Design review of the part built by this model. Coordinates are the model's own, in mm. Face numbers are marked on the shaded views. A direction names the side the tool comes from. Round coordinates to 2 decimals unless told otherwise and drop trailing zeros. Write each loop counter-clockwise with the first axis right and the second up, starting at its lowest first coordinate (ties: lowest second). Pieces come first, ordered by that corner, then holes. Notation, with made-up numbers: (87, 83) -> (146, 83) arc R11 cw to (146, 94) -> close; hole circle Ø5 at (-18, 79.5). An arc over 180 degrees is marked (long way). Write item = value, one per line. Start each with the question number.
Item 1: For pin 1 Ø2 at (y, z) = (-13, 7.5) entering from +X; pin 2 Ø1.5 at (y, z) = (7.5, 10.5) entering from +X; pin 3 Ø20 at (y, z) = (-1.5, 29) entering from -X, all flat-tipped, find the tip position at first contact; note any pin that passes through.
Item 2: Machinability: for the marked faces 1, 2 and 3, which of the approach directions +Z, -Z, +X, -X, +Y, -Y give a long, thin tool a straight path to every point of the face, cutting with its end or side? Answer none if there is none.
Item 3: To check wall thickness, follow L1, parallel to Y at x = -23.5, z = 33; L2, parallel to Y at x = -42, z = 19; L3, parallel to X at y = 3.5, z = 19. State the ranges of each line that lie inside material, in increasing order.
Item 4: Add section C-C, the plane y = 27. State the section outline as (x, z) points, then the cut area to 3 significant figures.
Item 5: Add section D-D, the plane x = -37. State the section outline as (y, z) points, then the cut area to 3 significant figures.
Item 6: Add section A-A, the plane z = 25. State the section outline as (x, y) points.
Item 7: Add section B-B, the plane x = -10. State the section outline as (y, z) points, then the cut area to 3 significant figures.
Item 8: Mouldability with a two-part tool opening along Z and no side actions: class the marked faces 4, 5 and 6 as released by +Z, released by -Z, zero draft, split by the parting line, or undercut.
from build123d import *

# Parameters (mm, degrees)
SKETCH_R        = 10
PAD_DEPTH       = 35
POCKET_DEPTH    = 70.001
CHAMFER_SIZE    = 20
CHAMFER001_SIZE = 20
SKETCH002_R     = 10
POCKET001_DEPTH = 15
SKETCH003_W     = 81.266709
SKETCH003_H     = 40
POCKET002_DEPTH = 65
SKETCH004_W     = 95.373383
SKETCH004_H     = 50
POCKET003_DEPTH = 20


with BuildPart() as part:
    # Sketch → Pad (new body, symmetric)
    with BuildSketch(Plane.XZ):
        with BuildLine():
            Line((50, 50), (50, 0))
            Line((50, 0), (-50, 0))
            Line((-50, 0), (-50, 30))
            ThreePointArc((-5.278546, 50), (-29.773495, 44.772275), (-50, 30))
            Line((50, 50), (-5.278546, 50))
        make_face()
        with Locations((-10, 25)):
            Circle(SKETCH_R, mode=Mode.SUBTRACT)
    extrude(amount=PAD_DEPTH, both=True)

    # Sketch001 → Pocket (cut, through all)
    with BuildSketch(Plane.XZ.offset(35)):
        Polygon((50, 50), (30, 50), (50, 38.452995), align=None)
        Polygon((50, 0), (30, 0), (50, 11.547005), align=None)
    extrude(amount=-POCKET_DEPTH, mode=Mode.SUBTRACT)

    # Chamfer
    chamfer_edges = [part.edges().sort_by_distance(p)[0] for p in [
        (50, -35, 25),
    ]]
    chamfer(chamfer_edges, length=CHAMFER_SIZE)

    # Chamfer001
    chamfer001_edges = [part.edges().sort_by_distance(p)[0] for p in [
        (50, 35, 25),
    ]]
    chamfer(chamfer001_edges, length=CHAMFER001_SIZE)

    # Sketch002 → Pocket001 (cut)
    with BuildSketch(Plane(origin=(50, 0, 0), x_dir=(0, 0, 1), z_dir=(1, 0, 0))):
        with Locations((25, 0)):
            Circle(SKETCH002_R)
    extrude(amount=-POCKET001_DEPTH, mode=Mode.SUBTRACT)

    # Sketch003 → Pocket002 (cut)
    with BuildSketch(Plane(origin=(-50, 0, 0), x_dir=(0, 0, -1), z_dir=(-1, 0, 0))):
        with Locations((-25.823334, 0)):
            Rectangle(SKETCH003_W, SKETCH003_H)
    extrude(amount=-POCKET002_DEPTH, mode=Mode.SUBTRACT)

    # Sketch004 → Pocket003 (cut)
    with BuildSketch(Plane(origin=(-50, 0, 0), x_dir=(0, 0, -1), z_dir=(-1, 0, 0))):
        with Locations((-23.676658, 0)):
            Rectangle(SKETCH004_W, SKETCH004_H)
    extrude(amount=-POCKET003_DEPTH, mode=Mode.SUBTRACT)


solid = part.part
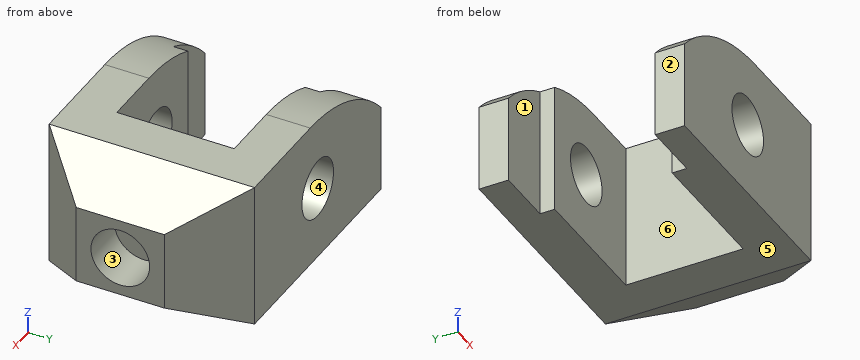
Result set:
q1.pin_1 = 44.72
q1.pin_2 = 49.49
q1.pin_3 = 15
q2.face_1 = +Z, -Z, -X
q2.face_2 = +Z, -Z, -X, +Y, -Y
q2.face_3 = +X
q3.L1 = -35 to -20, 20 to 35
q3.L2 = -35 to -25, 25 to 35
q3.L3 = 15 to 35
q4.outline = (-50, 0) -> (30, 0) -> (38, 4.62) -> (38, 45.38) -> (30, 50) -> (-5.28, 50) arc R60 ccw to (-50, 30) -> close; hole circle Ø20 at (-10, 25)
q4.area = 3,770 mm²
q5.outline = (-35, 0) -> (-25, 0) -> (-25, 40.93) -> (-35, 40.93) -> close; (25, 0) -> (35, 0) -> (35, 40.93) -> (25, 40.93) -> close
q5.area = 819 mm²
q6.outline = (-50, -35) -> (-20, -35) -> (-20, -20) -> (-30, -20) -> (-30, -25) -> (-50, -25) -> close; (-50, 25) -> (-30, 25) -> (-30, 20) -> (-20, 20) -> (-20, 35) -> (-50, 35) -> close; (0, -35) -> (30, -35) -> (50, -15) -> (50, -10) -> (35, -10) -> (35, 10) -> (50, 10) -> (50, 15) -> (30, 35) -> (0, 35) -> (0, 20) -> (15, 20) -> (15, -20) -> (0, -20) -> close
q7.outline = (-35, 0) -> (-20, 0) -> (-20, 15) -> (-35, 15) -> close; (-35, 35) -> (-20, 35) -> (-20, 49.81) -> (-35, 49.81) -> close; (20, 0) -> (35, 0) -> (35, 15) -> (20, 15) -> close; (20, 35) -> (35, 35) -> (35, 49.81) -> (20, 49.81) -> close
q7.area = 894 mm²
q8.face_4 = undercut
q8.face_5 = released by -Z
q8.face_6 = zero draft
